Geometry: see drawing. Coordinates: mm, zero at the bounding-box minimum. Coordinates: 2 decimals unless noted, no trailing zeros. Order: outer loops, then holes, each group sorted by start corner. A loop starts at its lowest first (then second) coordinate and runs counter-clockwise, first axis right, second up.
Item 1: Section B-B on y = 11. Return the cut outline in (x, z).
Item 2: Section C-C on x = 1.7. Return the cut outline in (y, z), then the cut area to 3 significant figures.
Item 3: Section A-A on z = 35.5. Return the cut outline in (x, y).
Item 4: Contact query for a flat-ended pin moving along its axis: P1, Ø1.6, axis at y = 39, z = 4.5, coming from the -X side. Output: stop coordinate, or through.
Item 5: Ray query, line 1 (Y direction, x = 1.2, z = 45.5) (1 decimal); line 2 (Z direction, x = 1.35, y = 10); line 3 (Y direction, x = 0.5, z = 32). Return the intervals inside material, ascending.
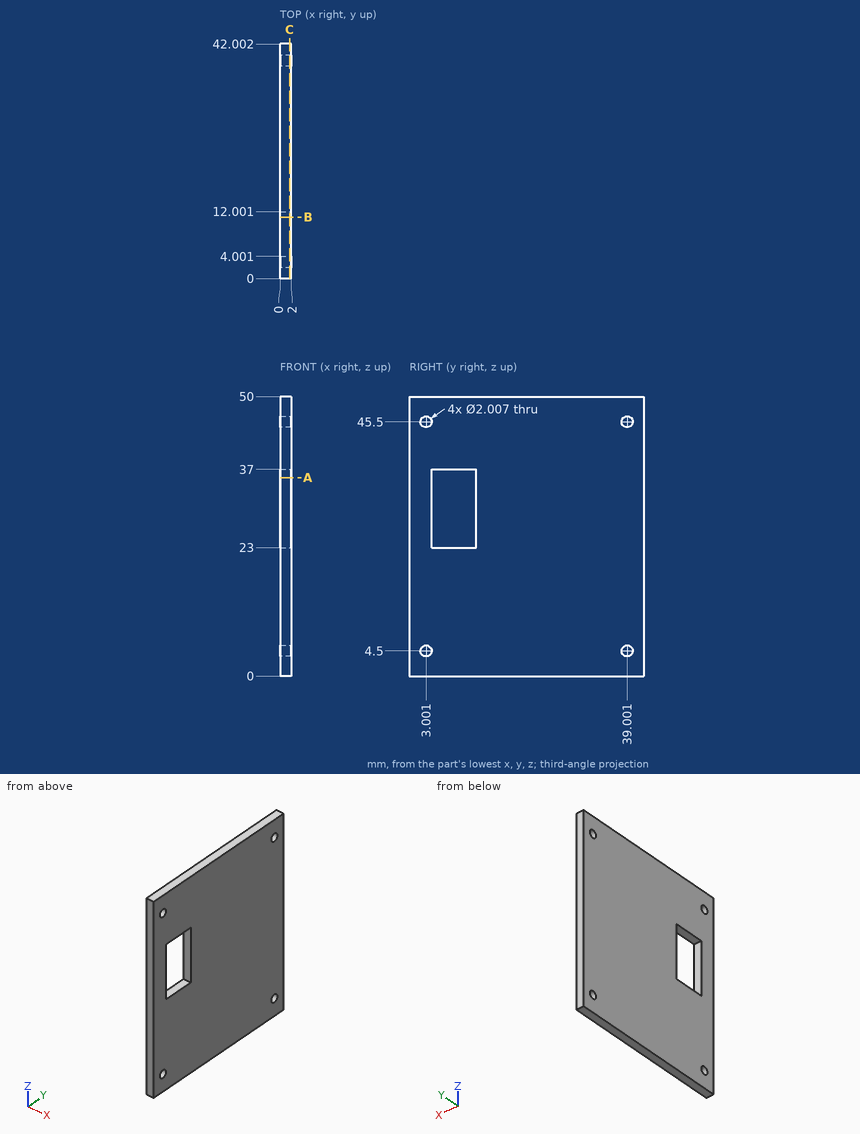
Answer list:
1. outline: (0, 0) - (2, 0) - (2, 23) - (0, 23) - close; (0, 37) - (2, 37) - (2, 50) - (0, 50) - close
2. outline: (0, 0) - (42, 0) - (42, 50) - (0, 50) - close; hole circle Ø2.01 at (3, 4.5); hole circle Ø2.01 at (3, 45.5); hole (4, 23) - (12, 23) - (12, 37) - (4, 37) - close; hole circle Ø2.01 at (39, 4.5); hole circle Ø2.01 at (39, 45.5)
2. area: 1,980 mm2
3. outline: (0, 0) - (2, 0) - (2, 4) - (0, 4) - close; (0, 12) - (2, 12) - (2, 42) - (0, 42) - close
4. P1: passes through
5. line 1: y = 0 to 2, 4 to 38, 40 to 42
5. line 2: z = 0 to 23, 37 to 50
5. line 3: y = 0 to 4, 12 to 42
